For this review, take the finished solid that the model builds, in its own axes (mm). A direction names the side the tool comes from. Give positions to 0.01 mm unless a question says otherwise; leave off trailing zeros. Order: outer loops, then holes, each group sorted by start corner. A loop starts at its lowest first (then second) coordinate and runs counter-clockwise, first axis right, second up. Notation, with made-up numbers: (-38, 45.25) - (-5, 45.25) arc R34 cw to (-5, 75.25) - close; hole circle Ø9 at (55, 67). An arc over 180 degrees is marked (long way). Use a Markdown table: item, result. Add a question column.
1) We need section B-B on x = 11.25. Write out the cut boundary in (y, z), then the cut area to 3 significant figures.
2) We need section C-C on y = 2.25. Give the number of separate pieces and of enclosed holes in the cut face, then the cut area to 3 significant figures.
3) Clearance check with flat-ended pins moving along their axes: P1, Ø0.9, axis at y = 4, z = -5, coming from the +X side; P2, Ø0.6, axis at y = 4.5, z = 1, coming from the -X side; P3, Ø0.9, axis at y = 4, z = 0.5, coming from the +X side; P4, Ø2, axis at x = 13.5, y = 2.25, coming from the +Z side. State where each tip first meets the part, or that it passes through.
4) Mouldability with a two-part tool opening along Y and no side actions: class faces 1 (the face through (12.63, 1.58, 0.04)), 2 (the face through (1, 2.3, 5.6)), 3 (the face through (12, 3, -3)), 4 (the face through (8, 0, 0)) as released by +Y, released by -Y, zero draft, split by the parting line, or undercut.
5) Machinability: for faces 5 (the face through (6, 3, 0)), 6 (the face through (5.7, 4.5, 0)), which of the approach directions +Z, -Z, +X, -X, +Y, -Y give a long, thin tool a straight path to every point of the face, cutting with its end or side? Answer none if there is none.
6) We need section D-D on z = 2. Write out the cut boundary in (x, y), then the cut area to 3 significant figures.
7) Wall thickness on L1, parallel to Y at x = 2, z = 4.85; L2, parallel to Z at x = 11.75, y = 4.1; L3, parallel to Z at x = 2.5, y = 3.55: over which ranges is each line inside the solid? List them lowest first.
8) We need section A-A on z = -6.5. Write out the cut boundary in (x, y).
```python
from build123d import *

# Parameters (mm, degrees)
GRUNDK_RPER_DEPTH         = 4.5
SKIZZE2_R                 = 1
SKIZZE2_R_2               = 1.1
ACHSBOHHRUNGEN_DEPTH      = 9
ACHSBOHHRUNGEN_DEPTH_BACK = 9
SKIZZE3_W                 = 2
SKIZZE3_H                 = 6.5
AUSSCHNITT_ZAHN_DEPTH     = 3
VERRUNDUNG2_R             = 2
FASE1_SIZE                = 0.3
FASE2_SIZE                = 0.3
MOOSGUMMIVERTIEFUNG_DEPTH = 0.8
VERRUNDUNG8_R             = 0.3


with BuildPart() as part:
    # Skizze1 → Grundkörper (new body)
    with BuildSketch(Plane(origin=(0, 0, 0), x_dir=(1, 0, 0), z_dir=(0, 1, 0))):
        Polygon((5.5, 3.25), (5.5, -3.25), (0, -3.25), (0, -8), (11, -8), (11, -3), (16, -3), (16, 3), (11, 3), (11, 8), (0, 8), (0, 3.25), align=None)
    extrude(amount=GRUNDK_RPER_DEPTH)

    # Skizze2 → Achsbohhrungen (cut, two sides)
    with BuildSketch(Plane.XY) as achsbohhrungen_sk:
        with Locations((2, 2.25)):
            Circle(SKIZZE2_R)
        with Locations((13.5, 2.25)):
            Circle(SKIZZE2_R_2)
    extrude(amount=ACHSBOHHRUNGEN_DEPTH, mode=Mode.SUBTRACT)
    extrude(achsbohhrungen_sk.sketch, amount=-ACHSBOHHRUNGEN_DEPTH_BACK, mode=Mode.SUBTRACT)

    # Skizze3 → Ausschnitt Zahn (cut)
    with BuildSketch(Plane.XZ):
        with Locations((6.5, 0)):
            Rectangle(SKIZZE3_W, SKIZZE3_H)
    extrude(amount=-AUSSCHNITT_ZAHN_DEPTH, mode=Mode.SUBTRACT)

    # Verrundung2
    verrundung2_edges = [part.edges().sort_by_distance(p)[0] for p in [
        (0, 0, -5.625),
        (16, 0, 0),
        (0, 0, 5.625),
        (16, 4.5, 0),
        (0, 4.5, -5.625),
        (0, 4.5, 5.625),
    ]]
    fillet(verrundung2_edges, radius=VERRUNDUNG2_R)

    # Fase1
    fase1_edges = [part.edges().sort_by_distance(p)[0] for p in [
        (11, 0, -5.5),
        (11, 4.5, 5.5),
        (11, 0, 5.5),
        (11, 4.5, -5.5),
    ]]
    chamfer(fase1_edges, length=FASE1_SIZE)

    # Fase2
    fase2_edges = [part.edges().sort_by_distance(p)[0] for p in [
        (1, 2.25, 3.25),
        (1, 2.25, -8),
        (1, 2.25, -3.25),
        (1, 2.25, 8),
        (12.4, 2.25, -3),
        (12.4, 2.25, 3),
    ]]
    chamfer(fase2_edges, length=FASE2_SIZE)

    # Skizze6 → MoosgummiVertiefung (cut)
    with BuildSketch(Plane(origin=(0, 4.5, 0), x_dir=(1, 0, 0), z_dir=(0, 1, 0))):
        Polygon((13.5, -2.5), (13.5, 2.5), (10.2, 2.5), (10.2, 7.5), (2.5, 7.5), (2.5, 3.75), (6, 3.75), (6, -3.75), (2.5, -3.75), (2.5, -7.5), (10.2, -7.5), (10.2, -2.5), align=None)
    extrude(amount=-MOOSGUMMIVERTIEFUNG_DEPTH, mode=Mode.SUBTRACT)

    # Verrundung8
    verrundung8_edges = [part.edges().sort_by_distance(p)[0] for p in [
        (13.5, 4.1, 2.5),
        (10.2, 4.1, 2.5),
        (10.2, 4.1, 7.5),
        (2.5, 4.1, 7.5),
        (2.5, 4.1, 3.75),
        (6, 4.1, 3.75),
        (6, 4.1, -3.75),
        (2.5, 4.1, -3.75),
        (2.5, 4.1, -7.5),
        (10.2, 4.1, -7.5),
        (10.2, 4.1, -2.5),
        (13.5, 4.1, -2.5),
    ]]
    fillet(verrundung8_edges, radius=VERRUNDUNG8_R)


solid = part.part
```
Checked values:
| question | item | result |
|---|---|---|
| 1 | outline | (0, -3) - (4.5, -3) - (4.5, -2.5) - (3.7, -2.5) - (3.7, 2.5) - (4.5, 2.5) - (4.5, 3) - (0, 3) - close |
| 1 | area | 23.0 mm² |
| 2 | separate pieces | 4 |
| 2 | enclosed holes | 0 |
| 2 | area | 125 mm² |
| 3 | P1 | x = 11 |
| 3 | P2 | x = 5.5 |
| 3 | P3 | x = 15.7 |
| 3 | P4 | through |
| 4 | face 1 | undercut |
| 4 | face 2 | undercut |
| 4 | face 3 | zero draft |
| 4 | face 4 | released by -Y |
| 5 | face 5 | -X, -Y |
| 5 | face 6 | +Z, -Z, +X, -X, +Y |
| 6 | outline | (5.5, 3) - (7.5, 3) - (7.5, 0) - (14, 0) arc R2 ccw to (16, 2) - (16, 2.5) arc R2 ccw to (14, 4.5) - (13.5, 4.5) - (13.5, 3.7) - (6, 3.7) - (6, 4.5) - (5.5, 4.5) - close; hole circle Ø2.2 at (13.5, 2.25) |
| 6 | area | 29.7 mm² |
| 7 | L1 | 0 to 1.25, 3.25 to 4.5 |
| 7 | L2 | -3 to -2.5, 2.5 to 3 |
| 7 | L3 | -8 to -3.25, 3.25 to 8 |
| 8 | outline | (0, 2) arc R2 ccw to (2, 0) - (10.7, 0) - (11, 0.3) - (11, 4.2) - (10.7, 4.5) - (10.2, 4.5) - (10.2, 3.7) - (2.5, 3.7) - (2.5, 4.5) - (2, 4.5) arc R2 ccw to (0, 2.5) - close; hole circle Ø2 at (2, 2.25) |
